Could you check a few things on this model? Use its own coordinates, in mm. A direction names the side the tool comes from. Coordinates: 2 decimals unless noted, no trailing zeros. Loops run counter-clockwise (first coordinate to the right, second up) from the corner with the lowest first, then second, coordinate; pieces in that order, holes last.
from build123d import *

# Parameters (mm, degrees)
SKETCH1_W           = 266.7
SKETCH1_H           = 172.72
BOSS_EXTRUDE1_DEPTH = 5.334
SKETCH2_W           = 38.1
SKETCH2_H           = 5.334
CUT_EXTRUDE1_DEPTH  = 165.701204222
SKETCH5_W           = 25.4
SKETCH5_H           = 6.096
SKETCH5_W_2         = 21.477624924
SKETCH5_W_3         = 21.477624925
CUT_EXTRUDE3_DEPTH  = 165.701204222
SKETCH9_W           = 5.334
SKETCH9_H           = 19.191111111
CUT_EXTRUDE7_DEPTH  = 165.701204222
SKETCH10_W          = 38.1
SKETCH10_H          = 5.334
BOSS_EXTRUDE2_DEPTH = 50.8
SKETCH11_W          = 6.604
SKETCH11_H          = 40.64
CUT_EXTRUDE8_DEPTH  = 197.710659379
SKETCH12_R          = 3.81
CUT_EXTRUDE9_DEPTH  = 197.710659379
SKETCH15_W          = 6.604
SKETCH15_H          = 10.16
CUT_EXTRUDE12_DEPTH = 197.710659379
SKETCH18_W          = 38.1
SKETCH18_H          = 56.134
BOSS_EXTRUDE3_DEPTH = 5.334
SKETCH19_W          = 34.756768033
SKETCH19_H          = 54.94363668
CUT_EXTRUDE15_DEPTH = 197.710659379
SKETCH21_R          = 0.889
CUT_EXTRUDE17_DEPTH = 197.710659379
SKETCH23_R          = 1.04775
CUT_EXTRUDE19_DEPTH = 197.710659379
SKETCH25_W          = 17.78
SKETCH25_H          = 5.334
CUT_EXTRUDE20_DEPTH = 197.710659379
SKETCH26_W          = 5.334
SKETCH26_H          = 12.7
CUT_EXTRUDE21_DEPTH = 197.710659379
SKETCH27_W          = 41.402
SKETCH27_H          = 48.26
CUT_EXTRUDE22_DEPTH = 197.710659379
SKETCH28_W          = 5.334
SKETCH28_H          = 22.86
CUT_EXTRUDE23_DEPTH = 197.710659379
SKETCH29_R          = 0.889
CUT_EXTRUDE24_DEPTH = 197.710659379
SKETCH30_W          = 2.032
SKETCH30_H          = 12.7
CUT_EXTRUDE25_DEPTH = 197.710659379


with BuildPart() as part:
    # Sketch1 → Boss-Extrude1 (new body)
    with BuildSketch(Plane.XY):
        with Locations((5.474099752, 2.104142138)):
            Rectangle(SKETCH1_W, SKETCH1_H)
    extrude(amount=BOSS_EXTRUDE1_DEPTH)

    # Sketch2 → Cut-Extrude1 (cut, through all)
    with BuildSketch(Plane.XY.offset(5.334)):
        with Locations((-70.725900248, -81.588857862)):
            Rectangle(SKETCH2_W, SKETCH2_H)
        with Locations((5.474099752, -81.588857862)):
            Rectangle(SKETCH2_W, SKETCH2_H)
        with Locations((81.674099752, -81.588857862)):
            Rectangle(SKETCH2_W, SKETCH2_H)
        with Locations((81.674099752, 85.797142138)):
            Rectangle(SKETCH2_W, SKETCH2_H)
        with Locations((5.474099752, 85.797142138)):
            Rectangle(SKETCH2_W, SKETCH2_H)
        with Locations((-70.725900248, 85.797142138)):
            Rectangle(SKETCH2_W, SKETCH2_H)
    extrude(amount=-CUT_EXTRUDE1_DEPTH, mode=Mode.SUBTRACT)

    # Sketch5 → Cut-Extrude3 (cut, through all)
    with BuildSketch(Plane.XY.offset(5.334)):
        with Locations((56.274099752, -26.343857862)):
            Rectangle(SKETCH5_W, SKETCH5_H)
        with Locations((-45.325900248, -26.343857862)):
            Rectangle(SKETCH5_W, SKETCH5_H)
        with Locations((-117.137087786, -26.343857862)):
            Rectangle(SKETCH5_W_2, SKETCH5_H)
        with Locations((128.08528729, -26.343857862)):
            Rectangle(SKETCH5_W_3, SKETCH5_H)
    extrude(amount=-CUT_EXTRUDE3_DEPTH, mode=Mode.SUBTRACT)

    # Sketch9 → Cut-Extrude7 (cut, through all)
    with BuildSketch(Plane.XY.offset(5.334)):
        with Locations((-125.208900248, -55.469191196)):
            Rectangle(SKETCH9_W, SKETCH9_H)
        with Locations((-125.208900248, -17.086968973)):
            Rectangle(SKETCH9_W, SKETCH9_H)
        with Locations((-125.208900248, 21.295253249)):
            Rectangle(SKETCH9_W, SKETCH9_H)
        with Locations((-125.208900248, 59.677475472)):
            Rectangle(SKETCH9_W, SKETCH9_H)
        with Locations((136.157099752, 59.677475472)):
            Rectangle(SKETCH9_W, SKETCH9_H)
        with Locations((136.157099752, 21.295253249)):
            Rectangle(SKETCH9_W, SKETCH9_H)
        with Locations((136.157099752, -17.086968973)):
            Rectangle(SKETCH9_W, SKETCH9_H)
        with Locations((136.157099752, -55.469191196)):
            Rectangle(SKETCH9_W, SKETCH9_H)
    extrude(amount=-CUT_EXTRUDE7_DEPTH, mode=Mode.SUBTRACT)

    # Sketch10 → Boss-Extrude2 (add)
    with BuildSketch(Plane(origin=(0, 88.464142138, 0), x_dir=(1, 0, 0), z_dir=(0, 1, 0))):
        with Locations((43.574099752, -2.667)):
            Rectangle(SKETCH10_W, SKETCH10_H)
    extrude(amount=BOSS_EXTRUDE2_DEPTH)

    # Sketch11 → Cut-Extrude8 (cut, through all)
    with BuildSketch(Plane(origin=(0, 0, 0), x_dir=(-1, 0, 0), z_dir=(0, 0, -1))):
        with Locations((-27.826099752, 108.784142138)):
            Rectangle(SKETCH11_W, SKETCH11_H)
    extrude(amount=-CUT_EXTRUDE8_DEPTH, mode=Mode.SUBTRACT)

    # Sketch12 → Cut-Extrude9 (cut, through all)
    with BuildSketch(Plane.XY.offset(5.334)):
        with Locations((43.574099752, 130.476471297)):
            Circle(SKETCH12_R)
    extrude(amount=-CUT_EXTRUDE9_DEPTH, mode=Mode.SUBTRACT)

    # Sketch15 → Cut-Extrude12 (cut, through all)
    with BuildSketch(Plane.XY.offset(5.334)):
        with Locations((27.826099752, 134.184142138)):
            Rectangle(SKETCH15_W, SKETCH15_H)
    extrude(amount=-CUT_EXTRUDE12_DEPTH, mode=Mode.SUBTRACT)

    # Sketch18 → Boss-Extrude3 (add)
    with BuildSketch(Plane.XY.offset(5.334)):
        with Locations((5.474099752, 111.197142138)):
            Rectangle(SKETCH18_W, SKETCH18_H)
    extrude(amount=-BOSS_EXTRUDE3_DEPTH)

    # Sketch19 → Cut-Extrude15 (cut, through all)
    with BuildSketch(Plane.XY.offset(5.334)):
        with Locations((48.506483768, 115.935960478)):
            Rectangle(SKETCH19_W, SKETCH19_H)
    extrude(amount=-CUT_EXTRUDE15_DEPTH, mode=Mode.SUBTRACT)

    # Sketch21 → Cut-Extrude17 (cut, through all)
    with BuildSketch(Plane.XY.offset(5.334)):
        with Locations((127.140099752, 59.677475471)):
            Circle(SKETCH21_R)
        with Locations(Location((-116.191900248, 59.677475471, 0), (0, 0, 180))):
            Circle(SKETCH21_R)
        with Locations((-116.191900248, -55.469191196)):
            Circle(SKETCH21_R)
        with Locations(Location((127.140099752, -55.469191196, 0), (0, 0, 180))):
            Circle(SKETCH21_R)
    extrude(amount=-CUT_EXTRUDE17_DEPTH, mode=Mode.SUBTRACT)

    # Sketch23 → Cut-Extrude19 (cut, through all)
    with BuildSketch(Plane(origin=(0, 0, 0), x_dir=(-1, 0, 0), z_dir=(0, 0, -1))):
        with Locations((-81.674099752, 75.510142138)):
            Circle(SKETCH23_R)
        with Locations(Location((70.725900248, 75.510142138, 0), (0, 0, 180))):
            Circle(SKETCH23_R)
    extrude(amount=-CUT_EXTRUDE19_DEPTH, mode=Mode.SUBTRACT)

    # Sketch25 → Cut-Extrude20 (cut, through all)
    with BuildSketch(Plane(origin=(0, 0, 0), x_dir=(-1, 0, 0), z_dir=(0, 0, -1))):
        with Locations((-117.869099752, -32.058857862)):
            Rectangle(SKETCH25_W, SKETCH25_H)
        with Locations((-82.309099752, -32.058857862)):
            Rectangle(SKETCH25_W, SKETCH25_H)
        with Locations((-46.749099752, -32.058857862)):
            Rectangle(SKETCH25_W, SKETCH25_H)
        with Locations((35.800900248, -32.058857862)):
            Rectangle(SKETCH25_W, SKETCH25_H)
        with Locations((106.920900248, -32.058857862)):
            Rectangle(SKETCH25_W, SKETCH25_H)
        with Locations((71.360900248, -32.058857862)):
            Rectangle(SKETCH25_W, SKETCH25_H)
    extrude(amount=-CUT_EXTRUDE20_DEPTH, mode=Mode.SUBTRACT)

    # Sketch26 → Cut-Extrude21 (cut, through all)
    with BuildSketch(Plane(origin=(0, 0, 0), x_dir=(-1, 0, 0), z_dir=(0, 0, -1))):
        with Locations((-82.309099752, -53.775857862)):
            Rectangle(SKETCH26_W, SKETCH26_H)
        with Locations((71.360900248, -53.775857862)):
            Rectangle(SKETCH26_W, SKETCH26_H)
    extrude(amount=-CUT_EXTRUDE21_DEPTH, mode=Mode.SUBTRACT)

    # Sketch27 → Cut-Extrude22 (cut, through all)
    with BuildSketch(Plane(origin=(0, 0, 0), x_dir=(-1, 0, 0), z_dir=(0, 0, -1))):
        with Locations((-5.474099752, -54.791857862)):
            Rectangle(SKETCH27_W, SKETCH27_H)
    extrude(amount=-CUT_EXTRUDE22_DEPTH, mode=Mode.SUBTRACT)

    # Sketch28 → Cut-Extrude23 (cut, through all)
    with BuildSketch(Plane(origin=(0, 0, 0), x_dir=(-1, 0, 0), z_dir=(0, 0, -1))):
        with Locations((-28.842099752, -44.631857862)):
            Rectangle(SKETCH28_W, SKETCH28_H)
        with Locations((-28.842099752, 1.088142138)):
            Rectangle(SKETCH28_W, SKETCH28_H)
        with Locations((-28.842099752, 46.808142138)):
            Rectangle(SKETCH28_W, SKETCH28_H)
        with Locations((17.893900248, 46.808142138)):
            Rectangle(SKETCH28_W, SKETCH28_H)
        with Locations((17.893900248, 1.088142138)):
            Rectangle(SKETCH28_W, SKETCH28_H)
        with Locations((17.893900248, -44.631857862)):
            Rectangle(SKETCH28_W, SKETCH28_H)
    extrude(amount=-CUT_EXTRUDE23_DEPTH, mode=Mode.SUBTRACT)

    # Sketch29 → Cut-Extrude24 (cut, through all)
    with BuildSketch(Plane(origin=(0, 0, 0), x_dir=(-1, 0, 0), z_dir=(0, 0, -1))):
        with Locations((-81.674099752, -75.111857862)):
            Circle(SKETCH29_R)
        with Locations(Location((70.725900248, -75.111857862, 0), (0, 0, 180))):
            Circle(SKETCH29_R)
    extrude(amount=-CUT_EXTRUDE24_DEPTH, mode=Mode.SUBTRACT)

    # Sketch30 → Cut-Extrude25 (cut, through all)
    with BuildSketch(Plane(origin=(0, 0, 0), x_dir=(-1, 0, 0), z_dir=(0, 0, -1))):
        with Locations((-5.474099752, 126.564142138)):
            Rectangle(SKETCH30_W, SKETCH30_H)
    extrude(amount=-CUT_EXTRUDE25_DEPTH, mode=Mode.SUBTRACT)


solid = part.part
1) Imagine slicing it at D-D on y = 20. List the corners of the cut face in (x, z) for me, plus the area to 3 significant figures.
2) Imagine slicing it at A-A on y = 42.5. List the corners of the cut face in (x, z) for me.
3) Will these pins go through, and if not, where does the flat tip stop? pin 1 (1 mm diameter, centred on x = -82, z = 1.5, fed in from +Y); pin 2 (1.6 mm diameter, centred on x = -38.5, z = 2, fed in from +Y); pin 3 (1.5 mm diameter, centred on x = -19.5, y = 49.5, fed in from -Z) (3 decimals); pin 4 (1.6 mm diameter, centred on x = -72.5, z = 1.5, fed in from -Y).
4) We'd pull the mould along X, two halves only. Please class faces 1 (the flat face through (118, -34.726, 3)), 2 (the flat face through (117.346, -26, 3)), 3 (the flat face through (55.639, -32, 3)), 4 (the flat face through (136, -7.491, 3)): released by +X, released by -X, zero draft, split by the parting line, or undercut.
5) If I drill on L1, parallel to X at y = 3, z = 4.2; L2, parallel to X at y = -75, z = 2; L3, parallel to X at y = -58, z = 4.6, over which ranges is the centre line in solid material (lowest first)?
6) Imagine slicing it at B-B on y = 114. List the corners of the cut face in (x, z) for me, plus the area to 3 significant figures.
7) For faces 5 (the flat face through (-109, -84.256, 3)), 6 (the flat face through (-32.626, -26, 3)), 7 (the flat face through (-125, 30.891, 3)), which set-ups out of +Z, -Z, +X, -X, +Y, -Y let a thin tool reach every point of the face, with its end or its side?
8) Imagine slicing it at C-C on z = 4.4. State how many separate pieces and enclosed holes the cut face has, plus the area to 3 significant figures.
Solved:
1. outline: (-122.54, 0) - (133.49, 0) - (133.49, 5.33) - (-122.54, 5.33) - close
1. area: 1,370 mm2
2. outline: (-127.88, 0) - (-20.56, 0) - (-20.56, 5.33) - (-127.88, 5.33) - close; (-15.23, 0) - (26.18, 0) - (26.18, 5.33) - (-15.23, 5.33) - close; (31.51, 0) - (138.82, 0) - (138.82, 5.33) - (31.51, 5.33) - close
3. pin 1: stops at y = 83.13
3. pin 2: stops at y = 88.46
3. pin 3: passes through
3. pin 4: stops at y = -78.92
4. face 1: undercut
4. face 2: released by +X
4. face 3: undercut
4. face 4: zero draft
5. L1: x = -127.88 to -20.56, -15.23 to 26.18, 31.51 to 138.82
5. L2: x = -127.88 to -71.61, -69.84 to -15.23, 26.18 to 80.79, 82.56 to 138.82
5. L3: x = -122.54 to -74.03, -68.69 to -15.23, 26.18 to 79.64, 84.98 to 133.49
6. outline: (-13.58, 0) - (24.52, 0) - (24.52, 5.33) - (-13.58, 5.33) - close
6. area: 203 mm2
7. face 5: +Z, -Z, +X, -X, -Y
7. face 6: +Z, -Z
7. face 7: +Z, -Z, -X
8. separate pieces: 1
8. enclosed holes: 19
8. area: 42,100 mm2
